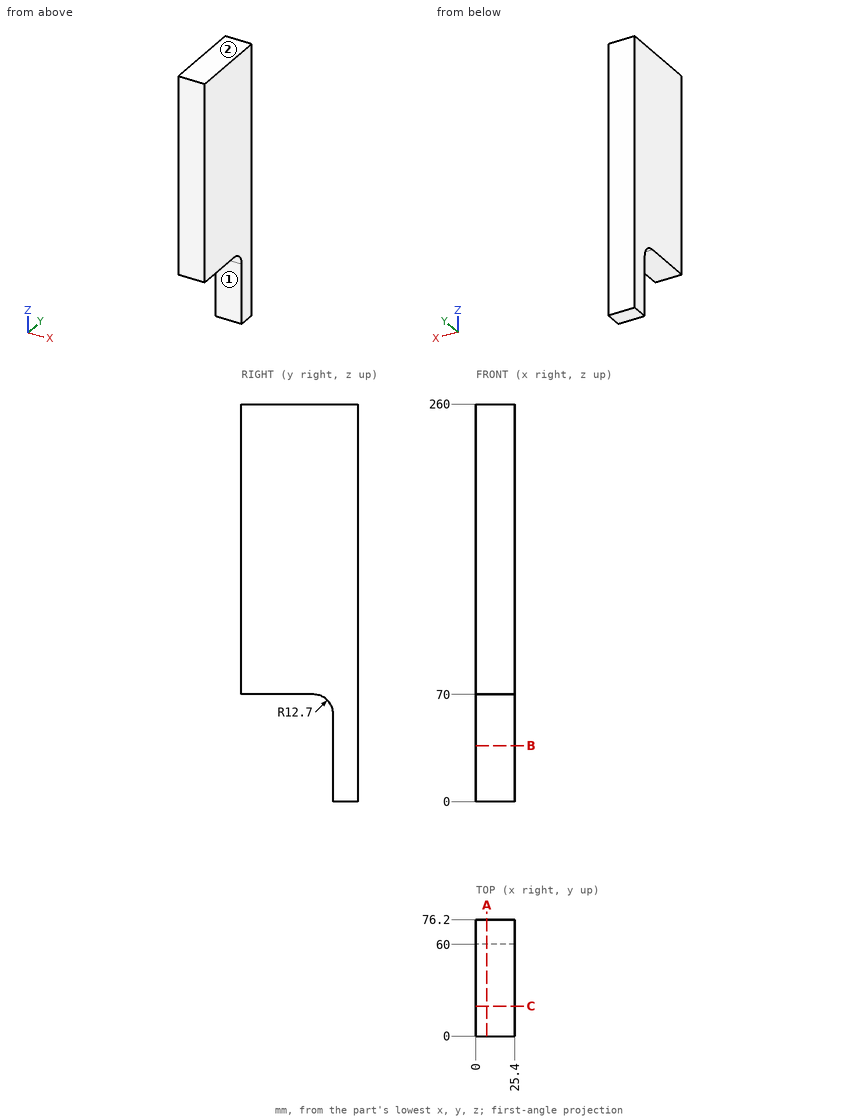
Source: three-view drawing plus pictorial views. Frame: mm from the lowest corner of the part. A direction names the side the tool comes from. Give positions to 0.01 mm unless a question says otherwise; leave off trailing zeros. Loops run counter-clockwise (first coordinate to the right, second up) from the corner with the lowest first, then second, coordinate; pieces in that order, holes last. Notation, with made-up numbers: M 4.5,48.5 L 58.5,48.5 A8 ccw 58.5,59.5 Z; hole C -17.75,80 d3. An arc over 180 degrees is marked long. Put each result on its own line as item: value.
Q1. Section A-A (x = 7.25). Return the cut outline in (y, z), and give its area (3 significant figures).
Response values:
outline: M 0,70 L 47.3,70 A12.7 cw 60,57.3 L 60,0 L 76.2,0 L 76.2,260 L 0,260 Z
area: 15,600 mm²
Q2. Section C-C (y = 19.5). Return the cut outline in (x, z), and give its area (3 significant figures).
Response values:
outline: M 0,70 L 25.4,70 L 25.4,260 L 0,260 Z
area: 4,830 mm²
Q3. Section B-B (z = 36.5). Return the cut outline in (x, y).
Response values:
outline: M 0,60 L 25.4,60 L 25.4,76.2 L 0,76.2 Z
Q4. Pin query (flat end, axial travel): P1, Ø8, axis at x = 11, y = 22.5, coming from the -Z side; P2, Ø6, axis at y = 67.5, z = 45.5, coming from the -X side; P3, Ø5, axis at x = 21, z = 34, coming from the -Y side; P4, Ø10, axis at x = 20, y = 49.5, coming from the -Z side. Return the tip coordinate at first contact, or that it passes through.
Response values:
P1: stops at z = 70
P2: stops at x = 0
P3: stops at y = 60
P4: stops at z = 67.76
Q5. Line query: probe 1 along Z at (x, y) = (14.75, 17); probe 2 along Z at (x, y) = (14.75, 53); probe 3 along Y at (x, z) = (16.5, 34). Output: solid intervals per line, ascending. Write a range as [from, to].
Response values:
probe 1: z = [70, 260]
probe 2: z = [68.65, 260]
probe 3: y = [60, 76.2]
Q6. Reachability of the marked faces 1 and 2 from +Z, -Z, +X, -X, +Y, -Y: full face, straight path, thin tool, end or side. Return the list, or none.
Response values:
face 1: -Z, +X, -X, -Y
face 2: +Z, +X, -X, +Y, -Y
